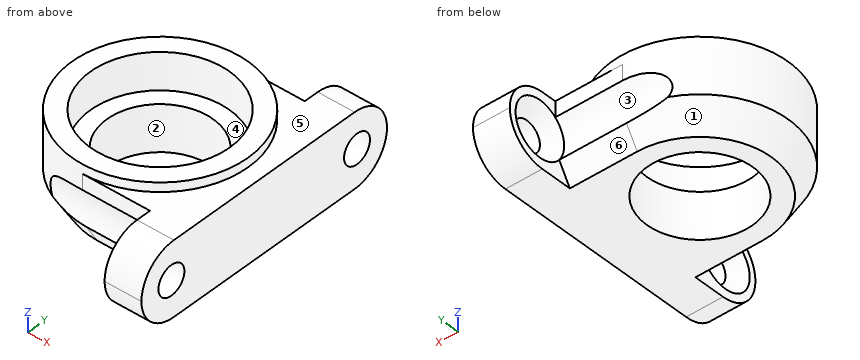
Autodesk Inventor part; units mm, degrees
ref_plane "РабПлоскость1" through (0, 0, 8) normal (0, 1, 0) x (1, 0, 0)
ref_plane "YZ Plane" through (0, 0, 0) normal (1, 0, 0) x (0, 1, 0)
ref_plane "XZ Plane" through (0, 0, 0) normal (0, 1, 0) x (-1, 0, 0)
sketch "Эскиз1" plane through (0, 0, 0) normal (0, 0, 1) x (1, 0, 0)
  circle A0 centre (0, 0) radius 5.75
  circle A1 centre (0, 0) radius 9.55
  dimension "d0" = 11.5
  dimension "d1" = 19.1
extrude "Выдавливание1" add sketch "Эскиз1" along normal blind 9
sketch "Эскиз2" plane through (0, 0, 9) normal (0, 0, 1) x (1, 0, 0)
  circle A0 centre (0, 0) radius 7.55
  dimension "d4" = 15.1
extrude "Выдавливание2" cut sketch "Эскиз2" against normal blind 4
chamfer "Фаска1" distance 3 distance2 1.8 1 edges at (-9.55, 0, 0) measured on face at (9.519, -0.7685, 6)
sketch "Эскиз3" plane through (0, 0, 0) normal (0, 0, -1) x (-1, 0, 0)
  circle A0 centre (0, 0) radius 5.75
  circle A1 centre (0, 0) radius 7.75
  circle A2 centre (0, 0) radius 9.55
  line L0 (0, 9.55) -> (-11.3, 9.55)
  line L1 (-11.3, 9.55) -> (-11.3, -9.55)
  line L2 (-11.3, -9.55) -> (0, -9.55)
  line L3 (0, -9.55) -> (0, 9.55)
  point P0 (0, -7.75)
  point P1 (0, 7.75)
  dimension "d10" = 11.3
extrude "Выдавливание3" add sketch "Эскиз3" against normal blind 8 contours A1 L3 A2 | A2 L2 L1 L0 picked at (-0.7618, -8.8575)
sketch "Эскиз4" plane through (0, 7.75, 0) normal (-1, 0, 0) x (0, 0, 1)
  line L0 (3, 1.8) -> (0, 0)
  line L1 (0, 1.8) -> (3, 1.8)
  line L2 (0, 0) -> (0, 1.8)
  line L3 (0, -17.3) -> (3, -17.3)
  line L4 (0, -15.5) -> (3, -17.3)
  line L5 (0, -17.3) -> (0, -15.5)
  line L6 (0, -17.3) -> (3, -17.3)
  point P0 (0, -7.75)
extrude "Выдавливание4" cut sketch "Эскиз4" against normal through all
sketch "Эскиз5" plane through (11.3, -9.55, 8) normal (1, 0, 0) x (0, 0, -1)
  line L0 (0, 19.1) -> (0, 0)
  line L1 (0, 19.1) -> (8, 19.1)
  line L2 (8, 19.1) -> (8, 24.7)
  line L3 (8, 24.7) -> (0, 24.7)
  line L4 (0, 24.7) -> (0, 19.1)
  line L5 (8, 19.1) -> (5, 19.1)
  line L6 (5, 19.1) -> (5, 16.7)
  line L7 (5, 16.7) -> (8, 16.7)
  line L8 (8, 16.7) -> (8, 19.1)
  line L9 (5, 0) -> (5, 19.1)
  point P0 (8, 9.55)
  dimension "d15" = 8
  dimension "d16" = 5.6
  dimension "d26" = 8
extrude "Выдавливание5" add sketch "Эскиз5" against normal blind 4
sketch "Эскиз6" plane through (7.3, -9.55, 8) normal (-1, 0, 0) x (0, 0, 1)
  line L0 (-5, 19.1) -> (-8, 17.3)
  line L1 (0, 19.1) -> (-5, 19.1)
  line L2 (0, 19.1) -> (0, 24.7)
  line L3 (0, 24.7) -> (-8, 24.7)
  line L4 (-8, 24.7) -> (-8, 17.3)
  line L5 (-8, 24.7) -> (-8, 17.3)
  line L6 (-8, 21) -> (0, 21)
  line L7 (0, 19.1) -> (0, 24.7)
  point P0 (-8, 9.55)
  point P1 (-4, 21)
hole "Отверстие1" at (7.3, 11.45, 4) direction (1, 0, 0) diameter 3.2 end through all countersink diameter 6 countersink angle 90
sketch "Эскиз8" plane through (7.3, -9.55, 8) normal (-1, 0, 0) x (0, 0, 1)
  arc A0 (-1.6784, 19.1) -> (-5.8148, 18.6111) centre (-4, 21) ccw
  circle A1 centre (-4, 21) radius 1.6
  arc A2 (-1.6784, 19.1) -> (-5.8148, 18.6111) centre (-4, 21) ccw
  arc A3 (-5.8148, 18.6111) -> (-1.6784, 19.1) centre (-4, 21) ccw
  circle A4 centre (-4, 21) radius 1.6
  point P0 (-8, 9.55)
  point P1 (-5.8148, 18.6111)
  point P2 (-1.6784, 19.1)
extrude "Выдавливание6" cut sketch "Эскиз8" along normal through all contours A3 A0 | A1
fillet "Сопряжение1" radius 4 2 edges at (9.3, 15.15, 0) (9.3, 15.15, 8)
ref_plane "РабПлоскость1" through (0, 0, 8) normal (0, 1, 0) x (1, 0, 0)
mirror "Зеркальное отражение1" about plane through (0, 0, 8) normal (0, 1, 0) of "Сопряжение1", "Отверстие1", "Выдавливание6", "Выдавливание5"
properties part number "Крепление дифференциала"
Design review of the part built by this model. Coordinates are the model's own, in mm. Face numbers are marked on the shaded views. A direction names the side the tool comes from. Round coordinates to 2 decimals unless told otherwise and drop trailing zeros. Write each loop counter-clockwise with the first axis right and the second up, starting at its lowest first coordinate (ties: lowest second). Pieces come first, ordered by that corner, then holes. Notation, with made-up numbers: (4, 5) -> (51, 5) arc R17 cw to (51, 31) -> close; hole circle Ø10 at (-7, 75.5). An arc over 180 degrees is marked (long way). One line per item, written item: value. Start each with the question number.
Q1. Insertion check: P1, Ø0.8, axis at x = 2.5, z = 7, coming from the +Y side; P2, Ø1.8, axis at x = 4, z = 7, coming from the -Y side; P3, Ø2, axis at x = 8.5, z = 3.5, coming from the +Y side; P4, Ø3.5, axis at y = -11.5, z = 6, coming from the -X side. Each pin has a flat end and moves straight along its axis. Give the tip position at first contact, or say it passes through.
Q2. The part is to be moulded in two halves that separate along X. For the marked faces 1, 2 and 3, say which applies: pulls with the +X half, pulls with the -X half, needs draft (parallel to the pull), parting line crosses it, or undercut.
Q3. Add section A-A (y = 0). Give the boundary of the cut face in (x, z).
Q4. Add section B-B (x = 3). Give the boundary of the cut face in (y, z).
Q5. Add section D-D (x = 6.5). Give the boundary of the cut face in (y, z).
Q6. Tool access review of the marked faces 4, 5 and 6: name each direction out of +Z, -Z, +X, -X, +Y, -Y from which nothing blocks a thin tool from reaching the whole face with its end or side.
Q7. To check wall thickness, follow probe 1 along Y at (x, z) = (9.95, 4); probe 2 along Y at (x, z) = (0, 7.3); probe 3 along Z at (x, y) = (10.75, -2). State the ranges of each line that lie inside material, in increasing order.
Q8. Add section C-C (z = 0.5). Give the boundary of the cut face in (x, y), then the cut area to 3 significant figures.
Response:
1. P1: stops at y = 9.55
1. P2: stops at y = -9.55
1. P3: stops at y = 15.15
1. P4: stops at x = 7.3
2. face 1: pulls with the -X half
2. face 2: undercut
2. face 3: needs draft
3. outline: (-9.55, 3) -> (-7.75, 0) -> (-5.75, 0) -> (-5.75, 5) -> (-7.55, 5) -> (-7.55, 9) -> (-9.55, 9) -> close; (5.75, 0) -> (11.3, 0) -> (11.3, 8) -> (9.55, 8) -> (9.55, 9) -> (7.55, 9) -> (7.55, 5) -> (5.75, 5) -> close
4. outline: (-9.55, 6.32) arc R3 cw to (-9.06, 2.19) -> (-7.75, 0) -> (-4.91, 0) -> (-4.91, 5) -> (-6.93, 5) -> (-6.93, 9) -> (-9.07, 9) -> (-9.07, 8) -> (-9.55, 8) -> close; (4.91, 0) -> (7.75, 0) -> (9.06, 2.19) arc R3 cw to (9.55, 6.32) -> (9.55, 8) -> (9.07, 8) -> (9.07, 9) -> (6.93, 9) -> (6.93, 5) -> (4.91, 5) -> close
5. outline: (-9.55, 6.32) arc R3 cw to (-9.06, 2.19) -> (-7.75, 0) -> (7.75, 0) -> (9.06, 2.19) arc R3 cw to (9.55, 6.32) -> (9.55, 8) -> (7, 8) -> (7, 9) -> (3.84, 9) -> (3.84, 5) -> (-3.84, 5) -> (-3.84, 9) -> (-7, 9) -> (-7, 8) -> (-9.55, 8) -> close
6. face 4: +Z
6. face 5: +Z, +X
6. face 6: -Z, -X, +Y
7. probe 1: y = -15.15 to -13.05, -9.85 to 9.85, 13.05 to 15.15
7. probe 2: y = -9.55 to -7.55, 7.55 to 9.55
7. probe 3: z = 0 to 8
8. outline: (0, -8.05) -> (7.3, -8.05) -> (7.3, -13.09) -> (11.3, -13.09) -> (11.3, 13.09) -> (7.3, 13.09) -> (7.3, 8.05) -> (0, 8.05) arc R8.05 ccw to start; hole circle Ø11.5 at (0, 0)
8. area: 220 mm^2
